Work out the finished part from the listing and answer in its coordinate system (mm). Coordinates: 2 decimals unless noted, no trailing zeros. Order: outer loops, then holes, each group sorted by start corner. A loop starts at its lowest first (then second) coordinate and runs counter-clockwise, first axis right, second up. Notation, with made-up numbers: (-23.75, -15.75) -> (30.25, -15.75) arc R15 ccw to (30.25, -5.75) -> close; hole circle Ø10 at (-36, 62.25). An arc over 180 degrees is marked (long way). Answer as CSV lines item,"result". Start each with the question number.
Item 1: Section C-C (x = -2.6) is taken. Write down the section's boundary in (y, z), then the cut area to 3 significant figures.
Item 2: Each of these flat-tipped pins is pushed along its axis until it touches: pin 1 Ø0.5 at (y, z) = (-2.5, 4) entering from +X; pin 2 Ø5 at (y, z) = (5.5, -2.5) entering from +X; pin 3 Ø3 at (x, z) = (0.5, -1) entering from -Y; pin 4 Ø0.6 at (y, z) = (-3, 1.5) entering from -X. Where does it stop, or does it pass through?
Item 3: Section B-B (y = 2.25) is taken. Write down the section's boundary in (x, z).
Item 4: For a pull along Z with two mould halves and no side action, classify faces 1 (the face through (0, 0, 0)), 2 (the face through (2.75, 4.69, 0.05)), 3 (the face through (-1, 6, 5)) as pulls with the +Z half, pulls with the -Z half, needs draft (parallel to the pull), parting line crosses it, or undercut.
Item 5: Straight lines are drawn through the part: L1, parallel to Z at x = -1.65, y = -1.5; L2, parallel to Y at x = -0.6, z = -3.75; L3, parallel to X at y = -1.5, z = -3.75. For each, find the intervals that lie inside material, in ascending order.
Item 6: Section D-D (z = 1.75) is taken. Write down the section's boundary in (x, y).
Item 7: Section A-A (y = -1.25) is taken. Write down the section's boundary in (x, z), then the cut area to 3 significant figures.
Autodesk Inventor part; units mm, degrees
ref_plane "YZ Plane" through (0, 0, 0) normal (1, 0, 0) x (0, 1, 0)
ref_plane "XZ Plane" through (0, 0, 0) normal (0, 1, 0) x (-1, 0, 0)
ref_plane "XY Plane" through (0, 0, 0) normal (0, 0, 1) x (1, 0, 0)
sketch "Sketch4" plane through (0, 0, 0) normal (1, 0, 0) x (0, 1, 0)
  line L0 (0, 0) -> (12, 0)
  line L1 (12, 0) -> (12, -2.75)
  line L2 (12, -2.75) -> (0, -2.75)
  line L3 (0, -2.75) -> (0, 0)
  line L4 (12, 0) -> (0, 0)
  line L5 (0, 0) -> (0, 2.75)
  line L6 (0, 2.75) -> (12, 2.75)
  line L7 (12, 2.75) -> (12, 0)
  circle A0 centre (9.25, 0) radius 2.75
  point P0 (9.25, 2.75)
  dimension "d7" = 12
  dimension "d8" = 2.75
  dimension "d9" = 12
  dimension "d10" = 2.75
revolve "Revolution1" add sketch "Sketch4" angle 360 about axis through (0, 0, 0) along (0, 1, 0) picked at (9.8215, 0.7167) contours L5 L6 A0 L0 | A0 L0
sketch "Sketch5" plane through (0, 0, 0) normal (0, -1, 0) x (1, 0, 0)
  circle A0 centre (0, 0) radius 2.75
  line L0 (0, 0) -> (1, 0)
  line L1 (1, 0) -> (1, 5)
  line L2 (1, 5) -> (-3, 5)
  line L3 (-3, 5) -> (-3, -5)
  line L4 (-3, -5) -> (1, -5)
  line L5 (1, -5) -> (1, 5)
  dimension "d12" = 1
  dimension "d13" = 5
  dimension "d14" = 4
  dimension "d15" = 10
extrude "Extrusion3" add sketch "Sketch5" against normal blind 12.5 contours L1 L5 A0 | A0 L5 L4 L3 L2 L1 picked at (-1.4731, -0.2204)
fillet "Fillet1" radius 0.1 8 edges at (1, 6.25, 5) (1, 12.5, 0) (-1, 12.5, 5) (-3, 12.5, 0) (1, 6.25, -5) (-1, 12.5, -5) (-3, 6.25, -5) (-3, 6.25, 5)
sketch "Sketch6" plane through (0, 0, 0) normal (0, -1, 0) x (1, 0, 0)
  line L0 (-3, -4.9) -> (-3, 4.9)
  line L1 (-1.8, 4.06) -> (-1.4, 4.06)
  line L2 (-1.4, 4.06) -> (-1.4, 3.56)
  line L3 (-1.4, 3.56) -> (-1.8, 3.56)
  line L4 (-1.8, 3.56) -> (-1.8, 4.06)
  line L5 (-1.8, 4.06) -> (-1.4, 3.56) construction
  line L6 (-1.4, 4.06) -> (-1.8, 3.56) construction
  line L7 (-1.8, -3.56) -> (-1.4, -3.56)
  line L8 (-1.4, -3.56) -> (-1.4, -4.06)
  line L9 (-1.4, -4.06) -> (-1.8, -4.06)
  line L10 (-1.8, -4.06) -> (-1.8, -3.56)
  line L11 (-1.8, -3.56) -> (-1.4, -4.06) construction
  line L12 (-1.4, -3.56) -> (-1.8, -4.06) construction
  line L13 (-1.8, 1.52) -> (-1.4, 1.52)
  line L14 (-1.4, 1.52) -> (-1.4, 1.02)
  line L15 (-1.4, 1.02) -> (-1.8, 1.02)
  line L16 (-1.8, 1.02) -> (-1.8, 1.52)
  line L17 (-1.8, 1.52) -> (-1.4, 1.02) construction
  line L18 (-1.4, 1.52) -> (-1.8, 1.02) construction
  point P0 (0, 0)
  dimension "d22" = 0.4
  dimension "d23" = 0.5
  dimension "d24" = 0.4
  dimension "d25" = 0.5
  dimension "d27" = 0.4
  dimension "d28" = 0.5
extrude "Extrusion4" add sketch "Sketch6" along normal blind 5
fillet "Fillet2" radius 0.5 12 edges at (-1.8, 0, 3.81) (-1.6, 0, 4.06) (-1.4, 0, 3.81) (-1.6, 0, 3.56) (-1.4, 0, 1.27) (-1.6, 0, 1.52) (-1.8, 0, 1.27) (-1.6, 0, 1.02) (-1.8, 0, -3.81) (-1.6, 0, -4.06) (-1.4, 0, -3.81) (-1.6, 0, -3.56)
properties part number "TSOP312"
Checked values:
1,outline,"(0, -5) -> (12.4, -5) arc R0.1 ccw to (12.5, -4.9) -> (12.5, 4.9) arc R0.1 ccw to (12.4, 5) -> (0, 5) -> close"
1,area,"125 mm^2"
2,pin 1,"stops at x = -1.4"
2,pin 2,"stops at x = 2.75"
2,pin 3,"stops at y = 0"
2,pin 4,"stops at x = -1.8"
3,outline,"(-3, -4.9) arc R0.1 ccw to (-2.9, -5) -> (0.9, -5) arc R0.1 ccw to (1, -4.9) -> (1, -2.56) arc R2.75 ccw to (1, 2.56) -> (1, 4.9) arc R0.1 ccw to (0.9, 5) -> (-2.9, 5) arc R0.1 ccw to (-3, 4.9) -> close"
4,face 1,"undercut"
4,face 2,"parting line crosses it"
4,face 3,"pulls with the +Z half"
5,L1,"z = -4.06 to -3.56, 1.02 to 1.52, 3.56 to 4.06"
5,L2,"y = 0 to 12.5"
5,L3,"x = -1.8 to -1.4"
6,outline,"(-3, 0) -> (-2.3, 0) arc R0.5 cw to (-2.03, -0.08) -> (-1.17, -0.08) arc R0.5 cw to (-0.9, 0) -> (2.12, 0) -> (2.12, 9.25) arc R2.12 ccw to (1, 11.12) -> (1, 12.4) arc R0.1 ccw to (0.9, 12.5) -> (-2.9, 12.5) arc R0.1 ccw to (-3, 12.4) -> close"
7,outline,"(-1.8, -4.06) -> (-1.4, -4.06) -> (-1.4, -3.56) -> (-1.8, -3.56) -> close; (-1.8, 1.02) -> (-1.4, 1.02) -> (-1.4, 1.52) -> (-1.8, 1.52) -> close; (-1.8, 3.56) -> (-1.4, 3.56) -> (-1.4, 4.06) -> (-1.8, 4.06) -> close"
7,area,"0.600 mm^2"
